Read the model definition and answer for the solid it produces. Units are mm, in the model's axes. A direction names the side the tool comes from. Give positions to 0.01 mm unless a question says otherwise; leave off trailing zeros. Write each loop counter-clockwise with the first axis right and the second up, starting at its lowest first coordinate (ties: lowest second). Pieces come first, ordered by that corner, then holes.
```python
from build123d import *

# Parameters (mm, degrees)
EXTRUDE_1_DEPTH      = 10
EXTRUDE_1_DEPTH_BACK = 10
CUT_EXTRUDE_1_DEPTH  = 5
EXTRUDE_2_DEPTH      = 0.5
SKETCH_4_R           = 6.5
EXTRUDE_3_DEPTH      = 1.5
SKETCH_5_R           = 2.95
EXTRUDE_4_DEPTH      = 4.2
FILLET_1_R           = 2
EXTRUDE_5_DEPTH      = 0.75


with BuildPart() as part:
    # Sketch 1 → Extrude 1 (new, two sides: drawn at the far end of the back side and taken through both)
    with BuildSketch(Plane.XY.offset(-EXTRUDE_1_DEPTH_BACK)):
        Polygon((-20.3, 19.95), (20.3, 19.95), (20.3, 12.05), (27.2, 12.05), (27.2, 9.55), (20.3, 9.55), (20.3, -19.95), (-20.3, -19.95), (-20.3, 9.55), (-27.2, 9.55), (-27.2, 12.05), (-20.3, 12.05), align=None)
    extrude(amount=EXTRUDE_1_DEPTH + EXTRUDE_1_DEPTH_BACK)

    # Sketch 2 → Cut-Extrude 1 (cut)
    with BuildSketch(Plane(origin=(0, 12.05, 0), x_dir=(1, 0, 0), z_dir=(0, 1, 0))):
        with BuildLine():
            Line((26.368211788, 4.25), (29.350265645, 4.25))
            Line((29.350265645, 4.25), (29.350265645, 5.75))
            Line((29.350265645, 5.75), (26.368211788, 5.75))
            ThreePointArc((26.368211788, 5.75), (22.1, 5), (26.368211788, 4.25))
        make_face()
        with BuildLine():
            Line((26.368211788, -4.25), (29.350265645, -4.25))
            Line((29.350265645, -4.25), (29.350265645, -5.75))
            Line((29.350265645, -5.75), (26.368211788, -5.75))
            ThreePointArc((26.368211788, -5.75), (22.1, -5), (26.368211788, -4.25))
        make_face()
        with BuildLine():
            Line((-26.368211788, -5.75), (-29.350265645, -5.75))
            Line((-29.350265645, -5.75), (-29.350265645, -4.25))
            Line((-29.350265645, -4.25), (-26.368211788, -4.25))
            ThreePointArc((-26.368211788, -4.25), (-22.1, -5), (-26.368211788, -5.75))
        make_face()
        with BuildLine():
            Line((-26.368211788, 4.25), (-29.350265645, 4.25))
            Line((-29.350265645, 4.25), (-29.350265645, 5.75))
            Line((-29.350265645, 5.75), (-26.368211788, 5.75))
            ThreePointArc((-26.368211788, 5.75), (-22.1, 5), (-26.368211788, 4.25))
        make_face()
    extrude(amount=-CUT_EXTRUDE_1_DEPTH, mode=Mode.SUBTRACT)

    # Sketch 3 → Extrude 2 (add)
    with BuildSketch(Plane(origin=(0, 19.95, 0), x_dir=(1, 0, 0), z_dir=(0, 1, 0))):
        with BuildLine():
            Line((-16.05, 8.4), (10.3, 8.4))
            ThreePointArc((10.3, 8.4), (18.7, 0), (10.3, -8.4))
            Line((10.3, -8.4), (-16.05, -8.4))
            ThreePointArc((-16.05, -8.4), (-16.757106781, -8.107106781), (-17.05, -7.4))
            Line((-17.05, -7.4), (-17.05, 7.4))
            ThreePointArc((-17.05, 7.4), (-16.757106781, 8.107106781), (-16.05, 8.4))
        make_face()
    extrude(amount=EXTRUDE_2_DEPTH)

    # Sketch 4 → Extrude 3 (add)
    with BuildSketch(Plane(origin=(0, 20.45, 0), x_dir=(1, 0, 0), z_dir=(0, 1, 0))):
        with Locations(Location((10.3, 0, 0), (0, 0, 90))):
            Circle(SKETCH_4_R)
    extrude(amount=EXTRUDE_3_DEPTH)

    # Sketch 5 → Extrude 4 (add)
    with BuildSketch(Plane(origin=(0, 21.95, 0), x_dir=(1, 0, 0), z_dir=(0, 1, 0))):
        with Locations(Location((10.3, 0, 0), (0, 0, 270))):
            Circle(SKETCH_5_R)
    extrude(amount=EXTRUDE_4_DEPTH)

    # Fillet 1
    fillet_1_edges = [part.edges().sort_by_distance(p)[0] for p in [
        (-27.2, 10.8, -10),
        (-27.2, 10.8, 10),
        (27.2, 10.8, 10),
        (27.2, 10.8, -10),
    ]]
    fillet(fillet_1_edges, radius=FILLET_1_R)

    # Sketch 8 → Extrude 5 (add, symmetric)
    with BuildSketch(Plane.XY):
        Polygon((20.3, 13.55), (20.3, 12.05), (25.3, 12.05), align=None)
    extrude_5 = extrude(amount=EXTRUDE_5_DEPTH, both=True)

    # Mirror 1: Extrude 5 across plane
    add(extrude_5.mirror(Plane(origin=(0, 0, 0), x_dir=(0, 0, 1), z_dir=(1, 0, 0))))


solid = part.part
```
Item 1: Section D-D (y = -6.5) is taken. Write down the section's boundary in (x, z).
Result set:
outline: (-20.3, -10) - (20.3, -10) - (20.3, 10) - (-20.3, 10) - close
Item 2: Find the intervals of material crossed by line 1 along Z through (x, y) = (-24.3, 11.55); line 2 along X through (y, z) = (16.5, -8.5); line 3 along X through (y, z) = (11.3, -5), in increasing order.
Result set:
line 1: z = -10 to -7.2, -2.8 to 2.8, 7.2 to 10
line 2: x = -20.3 to 20.3
line 3: x = -22.1 to 22.1
Item 3: Each of these flat-tipped pins is pushed along its axis until it touches: pin 1 Ø2.5 at (x, z) = (24.3, 5) entering from -Y; pin 2 Ø1.6 at (x, y) = (23.5, 13) entering from +Z; pin 3 Ø5.5 at (x, z) = (-24.5, 0) entering from +Y (3 decimals); pin 4 Ø0.6 at (y, z) = (20, -1) entering from -X. Where does it stop, or does it pass through?
Result set:
pin 1: passes through
pin 2: stops at z = 0.75
pin 3: stops at y = 13.115
pin 4: stops at x = -20.3
Item 4: Section C-C (x = -11) is taken. Write down the section's boundary in (y, z), and give its area (3 significant figures).
Result set:
outline: (-19.95, -10) - (19.95, -10) - (19.95, -8.4) - (20.45, -8.4) - (20.45, 8.4) - (19.95, 8.4) - (19.95, 10) - (-19.95, 10) - close
area: 806 mm2
Item 5: Section A-A (x = 24.3) is taken. Write down the section's boundary in (y, z).
Result set:
outline: (9.55, -10) - (12.05, -10) - (12.05, -7.2) - (9.55, -7.2) - close; (9.55, -2.8) - (12.05, -2.8) - (12.05, -0.75) - (12.35, -0.75) - (12.35, 0.75) - (12.05, 0.75) - (12.05, 2.8) - (9.55, 2.8) - close; (9.55, 7.2) - (12.05, 7.2) - (12.05, 10) - (9.55, 10) - close
Item 6: Determine the mould class of faces 5 (the cylindrical face through (-22.1, 10.82, 4.91)), 6 (the cylindrical face through (22.1, 10.82, 5.09)), 7 (the flat face through (24, 9.55, 0)), 8 (the flat face through (-20.3, -5, 0)) for opening direction X: pulls with the +X half, pulls with the -X half, needs draft (parallel to the pull), parting line crosses it, or undercut.
Result set:
face 5: undercut
face 6: undercut
face 7: needs draft
face 8: pulls with the -X half
Item 7: Which of the six approach directions +Z, -Z, +X, -X, +Y, -Y give full straight-line access (tool end or side, diameter ignored) to faces 1 (the flat face through (-21.7, 12.5, -0.75)), 2 (the cylindrical face through (14.255, 21.19, 5.158)), 3 (the cylindrical face through (18.7, 20.2, -0.18)), 4 (the flat face through (21.7, 12.5, 0.75))?
Result set:
face 1: -Z, -X, +Y
face 2: +Y
face 3: +X, +Y
face 4: +Z, +X, +Y
Item 8: Section B-B (z = 0) is taken. Write down the section's boundary in (x, y).
Result set:
outline: (-27.2, 9.55) - (-20.3, 9.55) - (-20.3, -19.95) - (20.3, -19.95) - (20.3, 9.55) - (27.2, 9.55) - (27.2, 12.05) - (25.3, 12.05) - (20.3, 13.55) - (20.3, 19.95) - (18.7, 19.95) - (18.7, 20.45) - (16.8, 20.45) - (16.8, 21.95) - (13.25, 21.95) - (13.25, 26.15) - (7.35, 26.15) - (7.35, 21.95) - (3.8, 21.95) - (3.8, 20.45) - (-17.05, 20.45) - (-17.05, 19.95) - (-20.3, 19.95) - (-20.3, 13.55) - (-25.3, 12.05) - (-27.2, 12.05) - close
